Part print with two shaded views. Sizes in mm from the minimum x, y, z corner. Give positions to 0.01 mm unless a question says otherwise; leave off trailing zeros. Order: outer loops, then holes, each group sorted by start corner. A loop starts at its lowest first (then second) coordinate and runs counter-clockwise, first axis right, second up. Notation, with made-up numbers: M 88.25,25 L 142.25,25 A14 cw 142.25,36 Z; hole C -33,67 d10. An arc over 180 degrees is marked long. Write each question's results on one line, items separated by ' | '. Start each with the question number.
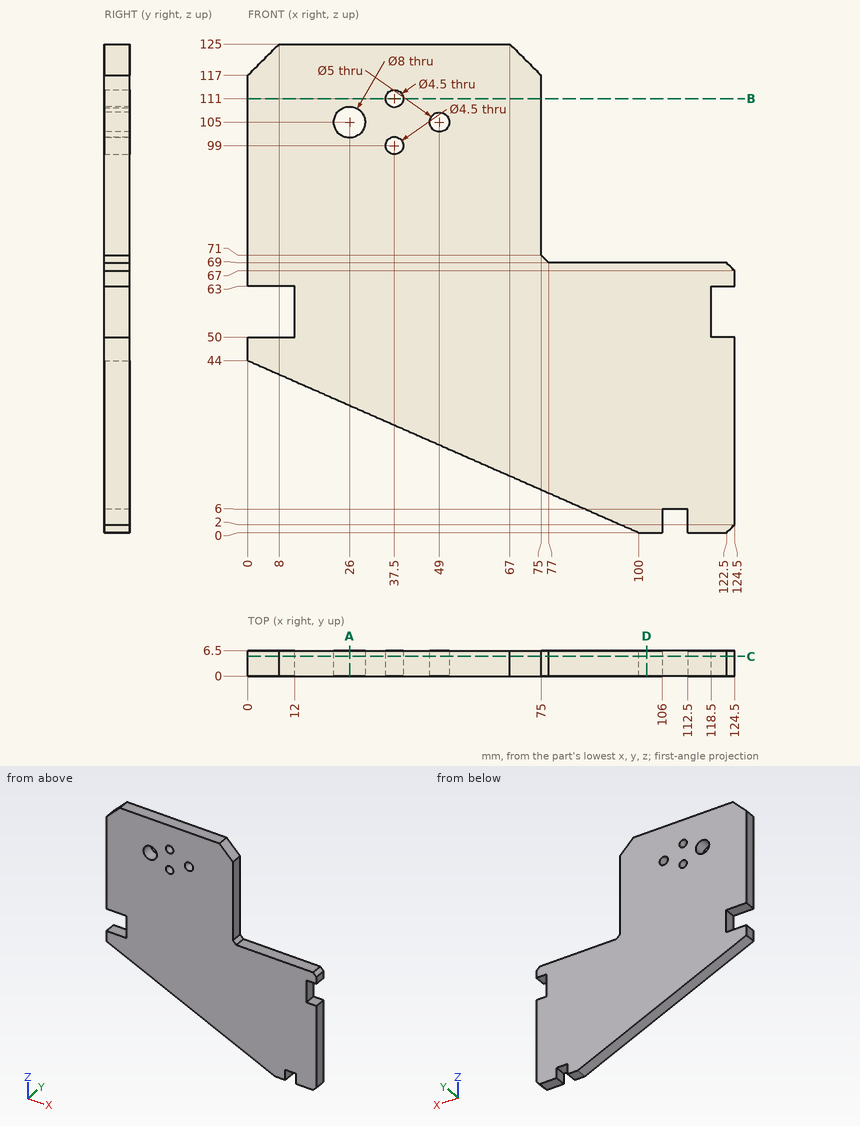
(1) Probe L1, parallel to X at y = 4.75, z = 99; L2, parallel to Z at x = 49, y = 2.25; L3, parallel to Z at x = 47, y = 4. List the from-to ranges inside material, lowest first.
(2) Saw through at D-D on x = 102. Give the cut face in (y, z).
(3) Saw through at A-A on x = 26. Give the cut face in (y, z).
(4) Drop flat-ended pins along their axis: P1, Ø2, axis at y = 4, z = 59, coming from the +X side; P2, Ø1, axis at y = 1, z = 52.5, coming from the -X side; P3, Ø3, axis at x = 67, y = 1, coming from the -Z side. Give the stop position or say it passes through.
(5) Saw through at C-C on y = 5. Give the cut face in (x, z).
(6) Saw through at B-B on z = 111. Give the cut face in (x, y), plus the area to 3 significant figures.
Taken from the geometry:
1) L1: x = 0 to 35.25, 39.75 to 75 | L2: z = 22.44 to 102.5, 107.5 to 125 | L3: z = 23.32 to 103.5, 106.5 to 125
2) outline: M 0,0 L 6.5,0 L 6.5,69 L 0,69 Z
3) outline: M 0,32.56 L 6.5,32.56 L 6.5,101 L 0,101 Z; M 0,109 L 6.5,109 L 6.5,125 L 0,125 Z
4) P1: stops at x = 118.5 | P2: stops at x = 12 | P3: stops at z = 13.86
5) outline: M 0,44 L 100,0 L 106,0 L 106,6 L 112.5,6 L 112.5,0 L 122.5,0 L 124.5,2 L 124.5,50 L 118.5,50 L 118.5,63 L 124.5,63 L 124.5,67 L 122.5,69 L 77,69 L 75,71 L 75,117 L 67,125 L 8,125 L 0,117 L 0,63 L 12,63 L 12,50 L 0,50 Z; hole C 26,105 d8; hole C 37.5,99 d4.5; hole C 37.5,111 d4.5; hole C 49,105 d5
6) outline: M 0,0 L 35.25,0 L 35.25,6.5 L 0,6.5 Z; M 39.75,0 L 75,0 L 75,6.5 L 39.75,6.5 Z | area: 458 mm²
